from build123d import *

# Parameters (mm, degrees)
F0_R     = 1.75
F1_DEPTH = 3
F2_SIZE2 = 2.8
F2_SIZE  = 1.6
F4_DEPTH = 0.2


with BuildPart() as f1:
    # F0 (on Top) → F1 (new body)
    with BuildSketch(Plane.XY):
        with BuildLine():
            Line((17.9, -39.193), (17.9, -44.793))
            ThreePointArc((17.9, -44.793), (22.9, -49.793), (27.9, -44.793))
            Line((27.9, -44.793), (27.9, -39.193))
            Line((27.9, -39.193), (39.6807047181, -39.193))
            Line((39.6807047181, -39.193), (50.1974673469, -49.6928583233))
            Line((50.1974673469, -49.6928583233), (68.6003446043, -49.6928583233))
            Line((68.6003446043, -49.6928583233), (68.6003446043, 33.6071416767))
            ThreePointArc((68.6003446043, 33.6071416767), (63.6003446043, 38.6071416767), (58.6003446043, 33.6071416767))
            Line((58.6003446043, 33.6071416767), (58.6003446043, 28.0071416767))
            Line((58.6003446043, 28.0071416767), (-0.1976553957, 28.0071416767))
            Line((-0.1976553957, 28.0071416767), (-0.1976553957, 33.6071416767))
            ThreePointArc((-0.1976553957, 33.6071416767), (-5.1976553957, 38.6071416767), (-10.1976553957, 33.6071416767))
            Line((-10.1976553957, 33.6071416767), (-10.1976553957, 10.6051872446))
            Line((-10.1976553957, 10.6051872446), (0.3, 0.124405442))
            Line((0.3, 0.124405442), (0.3, -39.193))
            Line((0.3, -39.193), (17.9, -39.193))
        make_face()
        with Locations((22.9, -44.793)):
            Circle(F0_R, mode=Mode.SUBTRACT)
        with Locations((-5.1976553957, 33.6071416767)):
            Circle(F0_R, mode=Mode.SUBTRACT)
        with Locations((63.6003446043, 33.6071416767)):
            Circle(F0_R, mode=Mode.SUBTRACT)
    extrude(amount=F1_DEPTH)

    # F2
    f2_edges = [f1.edges().sort_by_distance(p)[0] for p in [
        (21.15, -44.793, 0),
        (-6.947655, 33.607142, 0),
        (61.850345, 33.607142, 0),
    ]]
    f2_side = f1.faces().sort_by_distance((33.388783, -5.784916, 0))[0]
    chamfer(f2_edges, length=F2_SIZE, length2=F2_SIZE2, reference=f2_side)

    # F3 (on face) → F4 (join)
    with BuildSketch(Plane.XY.offset(3)):
        with BuildLine():
            ThreePointArc((4.8023446043, 33.6071416767), (-5.1976553957, 43.6071416767), (-15.1976553957, 33.6071416767))
            Line((-15.1976553957, 33.6071416767), (-15.1976553957, 10.6051872446))
            ThreePointArc((-15.1976553957, 10.6051872446), (-14.8162831751, 8.6899124771), (-13.7303444218, 7.0668107461))
            Line((-13.7303444218, 7.0668107461), (-4.7, -1.949018591))
            Line((-4.7, -1.949018591), (-4.7, -39.193))
            ThreePointArc((-4.7, -39.193), (-3.2355339059, -42.7285339059), (0.3, -44.193))
            Line((0.3, -44.193), (12.9, -44.193))
            Line((12.9, -44.193), (12.9, -44.793))
            ThreePointArc((12.9, -44.793), (23.2001352131, -54.7884949279), (32.8819837708, -44.193))
            Line((32.8819837708, -44.193), (37.6119923424, -44.193))
            Line((37.6119923424, -44.193), (46.6647783208, -53.2312348218))
            ThreePointArc((46.6647783208, -53.2312348218), (48.2859081001, -54.3130251219), (50.1974673469, -54.6928583233))
            Line((50.1974673469, -54.6928583233), (68.6003446043, -54.6928583233))
            ThreePointArc((68.6003446043, -54.6928583233), (72.1358785102, -53.2283922293), (73.6003446043, -49.6928583233))
            Line((73.6003446043, -49.6928583233), (73.6003446043, 33.6071416767))
            ThreePointArc((73.6003446043, 33.6071416767), (63.6003446043, 43.6071416767), (53.6003446043, 33.6071416767))
            Line((53.6003446043, 33.6071416767), (53.6003446043, 33.0071416767))
            Line((53.6003446043, 33.0071416767), (4.8023446043, 33.0071416767))
            Line((4.8023446043, 33.0071416767), (4.8023446043, 33.6071416767))
        make_face()
        with BuildLine():
            Line((0.3, 0.124405442), (-10.1976553957, 10.6051872446))
            Line((-10.1976553957, 10.6051872446), (-10.1976553957, 33.6071416767))
            ThreePointArc((-10.1976553957, 33.6071416767), (-5.1976553957, 38.6071416767), (-0.1976553957, 33.6071416767))
            Line((-0.1976553957, 33.6071416767), (-0.1976553957, 28.0071416767))
            Line((-0.1976553957, 28.0071416767), (58.6003446043, 28.0071416767))
            Line((58.6003446043, 28.0071416767), (58.6003446043, 33.6071416767))
            ThreePointArc((58.6003446043, 33.6071416767), (63.6003446043, 38.6071416767), (68.6003446043, 33.6071416767))
            Line((68.6003446043, 33.6071416767), (68.6003446043, -49.6928583233))
            Line((68.6003446043, -49.6928583233), (50.1974673469, -49.6928583233))
            Line((50.1974673469, -49.6928583233), (39.6807047181, -39.193))
            Line((39.6807047181, -39.193), (27.9, -39.193))
            Line((27.9, -39.193), (27.9, -44.793))
            ThreePointArc((27.9, -44.793), (22.9, -49.793), (17.9, -44.793))
            Line((17.9, -44.793), (17.9, -39.193))
            Line((17.9, -39.193), (0.3, -39.193))
            Line((0.3, -39.193), (0.3, 0.124405442))
        make_face(mode=Mode.SUBTRACT)
    extrude(amount=-F4_DEPTH)


solid = f1.part
Input: part model. Units: mm. Frame: model coordinates. A direction names the side the tool comes from. Give positions to 0.01 mm unless a question says otherwise; leave off trailing zeros. Loops run counter-clockwise (first coordinate to the right, second up) from the corner with the lowest first, then second, coordinate; pieces in that order, holes last. Notation, with made-up numbers: (71, -33.75) - (98, -33.75) arc R26 cw to (98, -18.75) - close; hole circle Ø1 at (81, 8). An arc over 180 degrees is marked (long way). Use CSV: the item, a comma, the result in double quotes. Start each with the question number.
Item 1: Section B-B on z = 1.5. Return loops of the section in (x, y), then the cut area to 3 significant figures.
Item 2: Line query: line 1 (X direction, y = 13.5, z = 0.4); line 2 (X direction, y = -39, z = 2.1); line 3 (Y direction, x = 32, z = 0.9). Output: solid intervals per line, ascending.
Item 3: Contact query for flat-ended pins moving along their axis: P1, Ø0.8, axis at x = 35, z = 1, coming from the +Y side; P2, Ø1.5, axis at x = 27, z = 1.5, coming from the -Y side; P3, Ø0.8, axis at y = -23.5, z = 1, coming from the +X side. Output: stop coordinate, or through.
Item 4: Section C-C on x = 36.5. Return loops of the section in (y, z), then the cut area to 3 significant figures.
Item 5: Section A-A on x = 22.9. Return loops of the section in (y, z), then the cut area to 3 significant figures.
Item 6: Mould query, pull axis Y, two halves, no side actions, for faces 6 (the cylindrical face through (-5.088, 38.606, 1.38)), 7 (the cylindrical face through (22.79, -49.79, 1.38)), 8 (the conical face through (65.29, 32.91, 2.66)), 9 (the flat face through (-0.198, 31, 1)). Classes: pulls with the +Y half, pulls with the -Y half, needs draft (parallel to the pull), parting line crosses it, or undercut.
Item 7: Reachability of faces 1 (the flat face through (68.6, -9, 1)), 2 (the flat face through (-5.022, 5.438, 1.38)), 3 (the flat face through (34, -39.193, 1)), 4 (the flat face through (58.6, 31, 1)), 5 (the flat face through (-1, -2, 2.8)) from +Z, -Z, +X, -X, +Y, -Y: full face, straight path, thin tool, end or side. Return the list, or none.
Ans:
1,outline,"(-10.2, 10.61) - (0.3, 0.12) - (0.3, -39.19) - (17.9, -39.19) - (17.9, -44.79) arc R5 ccw to (27.9, -44.79) - (27.9, -39.19) - (39.68, -39.19) - (50.2, -49.69) - (68.6, -49.69) - (68.6, 33.61) arc R5 ccw to (58.6, 33.61) - (58.6, 28.01) - (-0.2, 28.01) - (-0.2, 33.61) arc R5 ccw to (-10.2, 33.61) - close; hole circle Ø4.99 at (-5.2, 33.61); hole circle Ø4.99 at (22.9, -44.79); hole circle Ø4.99 at (63.6, 33.61)"
1,area,"5,300 mm2"
2,line 1,"x = -10.2 to 68.6"
2,line 2,"x = 0.3 to 68.6"
2,line 3,"y = -39.19 to 28.01"
3,P1,"stops at y = 28.01"
3,P2,"stops at y = -48.5"
3,P3,"stops at x = 68.6"
4,outline,"(-44.19, 2.8) - (-39.19, 2.8) - (-39.19, 0) - (28.01, 0) - (28.01, 2.8) - (33.01, 2.8) - (33.01, 3) - (-44.19, 3) - close"
4,area,"204 mm2"
5,outline,"(-54.79, 2.8) - (-49.79, 2.8) - (-49.79, 0) - (-48.14, 0) - (-46.54, 2.8) - (-46.54, 3) - (-54.79, 3) - close; (-43.04, 2.8) - (-41.44, 0) - (28.01, 0) - (28.01, 2.8) - (33.01, 2.8) - (33.01, 3) - (-43.04, 3) - close"
5,area,"220 mm2"
6,face 6,"pulls with the +Y half"
6,face 7,"pulls with the -Y half"
6,face 8,"undercut"
6,face 9,"needs draft"
7,face 1,"-Z, +X, +Y, -Y"
7,face 2,"-Z, -X, -Y"
7,face 3,"-Z, -Y"
7,face 4,"-Z, +Y"
7,face 5,"-Z"
